The listing builds one solid part. Answer for the finished solid, in the listing's coordinates (mm). A direction names the side the tool comes from. Coordinates: 2 decimals unless noted, no trailing zeros. Loops run counter-clockwise (first coordinate to the right, second up) from the corner with the lowest first, then second, coordinate; pieces in that order, holes last. Notation, with made-up numbers: M 8,0 L 50,0 A37 ccw 50,37 Z; hole C 16.5,31.5 d11. An arc over 180 degrees is marked long. Return JSON: item names as keys, results as strings. Group by question number.
1. Straight lines are drawn through the part: L1, parallel to X at y = -1.5, z = 1.95 (3 decimals); L2, parallel to Y at x = 13.65, z = 0.55; L3, parallel to Y at x = -16, z = 2. For each, find the intervals that lie inside material, in ascending order. Write a range as from..to.
2. Given P1, Ø4.5, axis at x = -13.65, y = 0, coming from the -Z side; P2, Ø2.5, axis at x = 13.65, y = 0, coming from the +Z side; P3, Ø1.6, axis at x = 14, y = 1, coming from the +Z side; P4, Ø1.5, axis at y = -1, z = 2.5, coming from the +X side, each flat-ended and moving along its own axis, determine where each tip first touches the part or whether it passes through.
3. Section B-B (x = -13.65) is taken. Write down the section's boundary in (y, z), then the cut area to 3 significant figures.
4. Which of the six approach directions +Z, -Z, +X, -X, +Y, -Y give full straight-line access (tool end or side, diameter ignored) to faces 1 (the face through (-12, -1, 1)), 2 (the face through (16, 3.57, 1.52))?
5. Section C-C (y = -1) is taken. Write down the section's boundary in (x, z), then the cut area to 3 significant figures.
6. The mould has two halves that part along Y. Classify faces 3 (the face through (-14.235, -2.636, 2.014)), 4 (the face through (0, 0, 0)), 5 (the face through (-16.07, 3.5, 1.52)), 6 (the face through (16.225, 0.811, 2.014)): pulls with the +Y half, pulls with the -Y half, needs draft (parallel to the pull), parting line crosses it, or undercut.
7. Section A-A (z = 0.4) is taken. Count the separate pieces of the cut face and the enclosed holes in it, then the cut area to 3 significant figures.
```python
from build123d import *

# Parameters (mm, degrees)
F0_W           = 35
F0_H           = 10
F0_W_2         = 20
F0_H_2         = 5
F1_DEPTH       = 3
F4_D           = 3
F4_CBORE_D     = 5.4
F4_CBORE_DEPTH = 2
F5_R           = 4.99999


# Not quite as in the source:
# - a fillet or chamfer is up to 0.001 mm smaller than in the source, because OpenCascade refuses the exact size


with BuildPart() as f1:
    # F0 (on Top) → F1 (new body)
    with BuildSketch(Plane.XY):
        Rectangle(F0_W, F0_H)
        Rectangle(F0_W_2, F0_H_2, mode=Mode.SUBTRACT)
        Rectangle(F0_W_2, F0_H_2)
    extrude(amount=F1_DEPTH)

    # F4 (through all)
    with Locations(Plane.XY.offset(3)):
        with Locations((-13.65, 0), (13.65, 0)):
            CounterBoreHole(F4_D / 2, F4_CBORE_D / 2, F4_CBORE_DEPTH)

    # F5 (radius 5 in the source; OpenCascade refuses exactly that, so slightly less here)
    f5_edges = [f1.edges().sort_by_distance(p)[0] for p in [
        (-17.5, -5, 1.5),
        (-17.5, 5, 1.5),
        (17.5, 5, 1.5),
        (17.5, -5, 1.5),
    ]]
    fillet(f5_edges, radius=F5_R)


solid = f1.part
```
Worked out:
{
 "1": {"L1": "-17.27..-15.895, -11.405..11.405, 15.895..17.27", "L2": "-4.87..-1.5, 1.5..4.87", "L3": "-3.57..-1.33, 1.33..3.57"},
 "2": {"P1": "z = 0", "P2": "through", "P3": "z = 1", "P4": "x = 17.49"},
 "3": {"outline": "M -4.87,0 L -1.5,0 L -1.5,1 L -2.7,1 L -2.7,3 L -4.87,3 Z; M 1.5,0 L 4.87,0 L 4.87,3 L 2.7,3 L 2.7,1 L 1.5,1 Z", "area": "15.4 mm^2"},
 "4": {"face 1": "+Z", "face 2": "+Z, -Z, +X, +Y"},
 "5": {"outline": "M -17.4,0 L -14.77,0 L -14.77,1 L -16.16,1 L -16.16,3 L -17.4,3 Z; M -12.53,0 L 12.53,0 L 12.53,1 L 11.14,1 L 11.14,3 L -11.14,3 L -11.14,1 L -12.53,1 Z; M 14.77,0 L 17.4,0 L 17.4,3 L 16.16,3 L 16.16,1 L 14.77,1 Z", "area": "79.9 mm^2"},
 "6": {"face 3": "undercut", "face 4": "needs draft", "face 5": "pulls with the +Y half", "face 6": "undercut"},
 "7": {"separate pieces": "1", "enclosed holes": "2", "area": "314 mm^2"}
}
